from build123d import *

# Parameters (mm, degrees)
SKETCH1_R               = 12
SKETCH1_R_2             = 3
BOSS_EXTRUDE1_DEPTH     = 4
SKETCH2_R               = 3.5
BOSS_EXTRUDE2_DEPTH     = 50.349572071
SKETCH3_W               = 2.224458382
SKETCH3_H               = 2.147670282
CUT_EXTRUDE1_DEPTH      = 4.436572991
CUT_EXTRUDE1_DEPTH_BACK = 100
SKETCH10_R              = 2.9
BOSS_EXTRUDE3_DEPTH     = 50


with BuildPart() as part:
    # Sketch1 → Boss-Extrude1 (new body)
    with BuildSketch(Plane(origin=(0, 0, 0), x_dir=(1, 0, 0), z_dir=(0, 1, 0))):
        Circle(SKETCH1_R)
        Circle(SKETCH1_R_2, mode=Mode.SUBTRACT)
        with BuildLine():
            Line((-2, -9.086626064), (-2, -5.913373936))
            ThreePointArc((-2, -5.913373936), (0, -3.913373936), (2, -5.913373936))
            Line((2, -5.913373936), (2, -9.086626064))
            ThreePointArc((2, -9.086626064), (0, -11.086626064), (-2, -9.086626064))
        make_face(mode=Mode.SUBTRACT)
        with BuildLine():
            Line((-9.086626064, 2), (-5.913373936, 2))
            ThreePointArc((-5.913373936, 2), (-3.913373936, 0), (-5.913373936, -2))
            Line((-5.913373936, -2), (-9.086626064, -2))
            ThreePointArc((-9.086626064, -2), (-11.086626064, 0), (-9.086626064, 2))
        make_face(mode=Mode.SUBTRACT)
        with BuildLine():
            Line((2, 9.086626064), (2, 5.913373936))
            ThreePointArc((2, 5.913373936), (0, 3.913373936), (-2, 5.913373936))
            Line((-2, 5.913373936), (-2, 9.086626064))
            ThreePointArc((-2, 9.086626064), (0, 11.086626064), (2, 9.086626064))
        make_face(mode=Mode.SUBTRACT)
        with BuildLine():
            Line((9.086626064, -2), (5.913373936, -2))
            ThreePointArc((5.913373936, -2), (3.913373936, 0), (5.913373936, 2))
            Line((5.913373936, 2), (9.086626064, 2))
            ThreePointArc((9.086626064, 2), (11.086626064, 0), (9.086626064, -2))
        make_face(mode=Mode.SUBTRACT)
        with BuildLine():
            Line((-5.255365036, -2.5), (-7.5, -2.5))
            Line((-7.5, -2.5), (-9.086626064, -2.5))
            ThreePointArc((-9.086626064, -2.5), (-10.071409475, -3.167974724), (-10.197041871, -4.351277348))
            ThreePointArc((-10.197041871, -4.351277348), (-7.780260231, -7.89815347), (-4.197441442, -10.261323639))
            ThreePointArc((-4.197441442, -10.261323639), (-3.073674879, -10.089196803), (-2.5, -9.107679575))
            Line((-2.5, -9.107679575), (-2.5, -7.5))
            Line((-2.5, -7.5), (-2.5, -5.256429725))
            Line((-2.5, -5.256429725), (-2.5, -5.255365036))
            ThreePointArc((-2.5, -5.255365036), (-3.303104097, -3.303104097), (-5.255365036, -2.5))
        make_face(mode=Mode.SUBTRACT)
        with BuildLine():
            Line((2.5, -5.255365036), (2.5, -7.5))
            Line((2.5, -7.5), (2.5, -9.086626064))
            ThreePointArc((2.5, -9.086626064), (3.167974724, -10.071409475), (4.351277348, -10.197041871))
            ThreePointArc((4.351277348, -10.197041871), (7.89815347, -7.780260231), (10.261323639, -4.197441442))
            ThreePointArc((10.261323639, -4.197441442), (10.089196803, -3.073674879), (9.107679575, -2.5))
            Line((9.107679575, -2.5), (7.5, -2.5))
            Line((7.5, -2.5), (5.256429725, -2.5))
            Line((5.256429725, -2.5), (5.255365036, -2.5))
            ThreePointArc((5.255365036, -2.5), (3.303104097, -3.303104097), (2.5, -5.255365036))
        make_face(mode=Mode.SUBTRACT)
        with BuildLine():
            Line((-2.5, 5.255365036), (-2.5, 7.5))
            Line((-2.5, 7.5), (-2.5, 9.086626064))
            ThreePointArc((-2.5, 9.086626064), (-3.167974724, 10.071409475), (-4.351277348, 10.197041871))
            ThreePointArc((-4.351277348, 10.197041871), (-7.89815347, 7.780260231), (-10.261323639, 4.197441442))
            ThreePointArc((-10.261323639, 4.197441442), (-10.089196803, 3.073674879), (-9.107679575, 2.5))
            Line((-9.107679575, 2.5), (-7.5, 2.5))
            Line((-7.5, 2.5), (-5.256429725, 2.5))
            Line((-5.256429725, 2.5), (-5.255365036, 2.5))
            ThreePointArc((-5.255365036, 2.5), (-3.303104097, 3.303104097), (-2.5, 5.255365036))
        make_face(mode=Mode.SUBTRACT)
        with BuildLine():
            Line((5.255365036, 2.5), (7.5, 2.5))
            Line((7.5, 2.5), (9.086626064, 2.5))
            ThreePointArc((9.086626064, 2.5), (10.071409475, 3.167974724), (10.197041871, 4.351277348))
            ThreePointArc((10.197041871, 4.351277348), (7.780260231, 7.89815347), (4.197441442, 10.261323639))
            ThreePointArc((4.197441442, 10.261323639), (3.073674879, 10.089196803), (2.5, 9.107679575))
            Line((2.5, 9.107679575), (2.5, 7.5))
            Line((2.5, 7.5), (2.5, 5.256429725))
            Line((2.5, 5.256429725), (2.5, 5.255365036))
            ThreePointArc((2.5, 5.255365036), (3.303104097, 3.303104097), (5.255365036, 2.5))
        make_face(mode=Mode.SUBTRACT)
    extrude(amount=BOSS_EXTRUDE1_DEPTH)

    # Sketch2 → Boss-Extrude2 (add)
    with BuildSketch(Plane(origin=(0, 4, 0), x_dir=(1, 0, 0), z_dir=(0, 1, 0))):
        Circle(SKETCH2_R)
    extrude(amount=BOSS_EXTRUDE2_DEPTH)

    # Sketch3 → Cut-Extrude1 (cut, two sides)
    with BuildSketch(Plane(origin=(0, 0, 0), x_dir=(0, 0, -1), z_dir=(1, 0, 0))) as cut_extrude1_sk:
        with Locations((0, 45.849702495)):
            Rectangle(SKETCH3_W, SKETCH3_H)
    extrude(amount=CUT_EXTRUDE1_DEPTH, mode=Mode.SUBTRACT)
    extrude(cut_extrude1_sk.sketch, amount=-CUT_EXTRUDE1_DEPTH_BACK, mode=Mode.SUBTRACT)

    # Sketch10 → Boss-Extrude3 (add)
    with BuildSketch(Plane(origin=(0, 54.349572071, 0), x_dir=(1, 0, 0), z_dir=(0, 1, 0))):
        Circle(SKETCH10_R)
    extrude(amount=BOSS_EXTRUDE3_DEPTH)


solid = part.part
Input: part model. Units: mm. Frame: model coordinates. A direction names the side the tool comes from. Coordinates: 2 decimals unless noted, no trailing zeros. Write each loop counter-clockwise with the first axis right and the second up, starting at its lowest first coordinate (ties: lowest second). Pieces come first, ordered by that corner, then holes. Notation, with made-up numbers: M 26,52 L 42,52 A4 ccw 42,56 Z; hole C 78,-27 d8. An arc over 180 degrees is marked long. Answer as a JSON object with one key per item and string values. Group by question number.
(1) Section C-C on y = 35.5. Output: boundary loops of the cut face in (x, z), plus the area to 3 significant figures.
(2) Contact query for flat-ended pins moving along their axis: P1, Ø2.5, axis at y = 2.5, z = 8, coming from the -X side; P2, Ø3, axis at x = 8, y = 2.5, coming from the -Z side; P3, Ø3, axis at y = 1.5, z = -7.5, coming from the -X side. Output: stop coordinate, or through.
(3) Ray query, line 1 along X through (y, z) = (1.45, 0); line 2 along Y through (x, z) = (9.75, -2.25). Return the intervals inside material, ascending. Write a range as [from, to].
(4) Mould query, pull axis Z, two halves, no side actions, for faces 1 (the face through (-2.9, 79, -0.1)), 2 (the face through (7, 2, -2)), 3 (the face through (-11.086, 1.972, 0.044)), 4 (the face through (1, 4, -4)). Classes: pulls with the +Z half, pulls with the -Z half, needs draft (parallel to the pull), parting line crosses it, or undercut.
(5) Section A-A on x = 0. Output: boundary loops of the cut face in (y, z).
(6) Set-up query: faces 5 (the face through (0, 46, -1.112)), 6 (the face through (-7.86, 1.97, -7.82)). Return all of +Z, -Z, +X, -X, +Y, -Y with unobstructed straight access to the full face (end or side cutting, diameter ignored); none if empty.
(7) Section D-D on y = 86.5. Output: boundary loops of the cut face in (x, z), plus the area to 3 significant figures.
(8) Section B-B on z = 0. Output: boundary loops of the cut face in (x, y).
Result set:
{
 "1": {"outline": "C 0,0 d7", "area": "38.5 mm2"},
 "2": {"P1": "stops at x = -9.92", "P2": "stops at z = -10.09", "P3": "stops at x = -10.39"},
 "3": {"line 1": "x = [-12, -11.09], [-3.91, -3], [3, 3.91], [11.09, 12]", "line 2": "y = [0, 4]"},
 "4": {"face 1": "parting line crosses it", "face 2": "undercut", "face 3": "undercut", "face 4": "needs draft"},
 "5": {"outline": "M 0,-12 L 4,-12 L 4,-11.09 L 0,-11.09 Z; M 0,-3.91 L 4,-3.91 L 4,-3.5 L 54.35,-3.5 L 54.35,-2.9 L 104.35,-2.9 L 104.35,2.9 L 54.35,2.9 L 54.35,3.5 L 4,3.5 L 4,3.91 L 0,3.91 L 0,3 L 4,3 L 4,-3 L 0,-3 Z; M 0,11.09 L 4,11.09 L 4,12 L 0,12 Z; hole M 44.78,-1.11 L 46.92,-1.11 L 46.92,1.11 L 44.78,1.11 Z"},
 "6": {"face 5": "+X, -X", "face 6": "+Y, -Y"},
 "7": {"outline": "C 0,0 d5.8", "area": "26.4 mm2"},
 "8": {"outline": "M -12,0 L -11.09,0 L -11.09,4 L -12,4 Z; M -3.91,0 L -3,0 L -3,4 L 3,4 L 3,0 L 3.91,0 L 3.91,4 L 3.5,4 L 3.5,44.78 L -3.5,44.78 L -3.5,4 L -3.91,4 Z; M -3.5,46.92 L 3.5,46.92 L 3.5,54.35 L 2.9,54.35 L 2.9,104.35 L -2.9,104.35 L -2.9,54.35 L -3.5,54.35 Z; M 11.09,0 L 12,0 L 12,4 L 11.09,4 Z"}
}
